```python
from build123d import *

# Parameters (mm, degrees)
F0_W      = 15.875
F0_H      = 15.875
F1_DEPTH  = 4.7625
F1_FACE_W = 15.875
F1_FACE_H = 15.875
F3_W      = 6.35
F3_H      = 6.35


with BuildPart() as f1:
    # F0 (on Top) → F1 (new body)
    with BuildSketch(Plane.XY):
        Rectangle(F0_W, F0_H)
    extrude(amount=F1_DEPTH)

    # F1_face (on face) → F4 section 0
    with BuildSketch(Plane.XY.offset(4.7625)):
        Rectangle(F1_FACE_W, F1_FACE_H)
    # F3 (on offset) → F4 section 1
    with BuildSketch(Plane.XY.offset(19.05)):
        Rectangle(F3_W, F3_H)
    loft()

    # F6 (on offset) → F7 (revolve)
    with BuildSketch(Plane.XY.offset(23.368)):
        with BuildLine():
            Line((0, -6.35), (0, 6.35))
            ThreePointArc((0, 6.35), (-6.35, 0), (0, -6.35))
        make_face()
    revolve(axis=Axis((0, 0, 23.368), (0, -1, 0)))


solid = f1.part
```
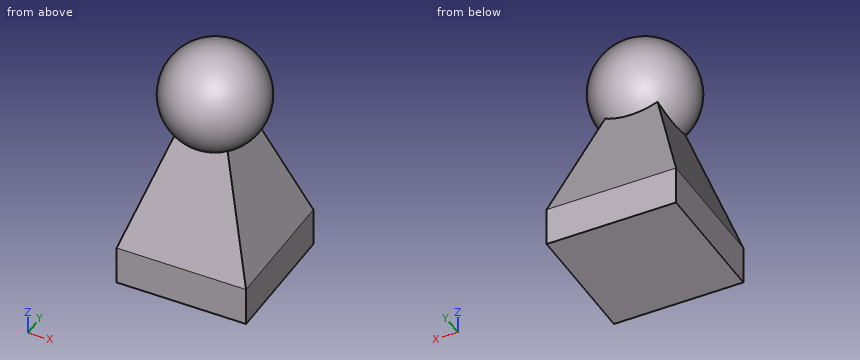
Part model, mm, in its own coordinate system. Coordinates: 2 decimals unless noted, no trailing zeros. Order: outer loops, then holes, each group sorted by start corner. A loop starts at its lowest first (then second) coordinate and runs counter-clockwise, first axis right, second up. Notation, with made-up numbers: (60.5, -16.75) -> (86.5, -16.75) arc R21 ccw to (86.5, 21.25) -> close; hole circle Ø10 at (-9.5, 39.25). An arc over 180 degrees is marked (long way). Put each result on its own line as item: value. Start each with the question number.
(1) Pin check, flat tips, straight feed: pin 1 Ø8 at (x, z) = (-2.5, 26) entering from +Y; pin 2 Ø4 at (x, z) = (4.5, 14) entering from +Y (3 decimals); pin 3 Ø6 at (x, z) = (6, 16.5) entering from -Y. Stop position of each tip, or through.
(2) Band-saw the part on B-B (z = 27). Give the cut face in (x, y), then the cut area to 3 significant figures.
(3) Band-saw the part on A-A (z = 20.75). Give the cut face in (x, y).
(4) Probe line 1 along Y through (x, z) = (-3.5, 15) (3 decimals); line 2 along Y through (x, z) = (2, 18.75); line 3 along Z through (x, y) = (-2.25, 3.25). List the from-to ranges inside material, lowest first. Write a range as [from, to].
Determined:
1. pin 1: stops at y = 6.35
1. pin 2: stops at y = 5.525
1. pin 3: stops at y = -4.96
2. outline: circle Ø10.42 at (0, 0)
2. area: 85.2 mm²
3. outline: circle Ø11.57 at (0, 0)
4. line 1: y = [-4.525, 4.525]
4. line 2: y = [-3.87, 3.87]
4. line 3: z = [0, 28.34]
